Could you check a few things on this model? Use its own coordinates, in mm. A direction names the side the tool comes from. Round coordinates to 2 decimals unless told otherwise and drop trailing zeros. Loops run counter-clockwise (first coordinate to the right, second up) from the corner with the lowest first, then second, coordinate; pieces in that order, holes last. Notation, with made-up numbers: (15.25, -4) - (47.25, -4) arc R25 ccw to (47.25, 32) - close; hole circle Ø2 at (13, 89.5). An arc over 180 degrees is marked (long way). Use one line per item in the form item = value.
```python
from build123d import *

# Parameters (mm, degrees)
SKETCH1_W           = 5.6
SKETCH1_H           = 10
BOSS_EXTRUDE1_DEPTH = 4.5
CHAMFER1_SIZE       = 1
SKETCH2_R           = 1.5
BOSS_EXTRUDE2_DEPTH = 0.9
SKETCH3_W           = 3.6
SKETCH3_H           = 0.5
BOSS_EXTRUDE3_DEPTH = 2.4
CHAMFER2_SIZE       = 0.5


# Read off the part's stored shape, not the designer's step: Dome1, Dome2
with BuildPart() as part:
    # Sketch1 → Boss-Extrude1 (new body)
    with BuildSketch(Plane.XY):
        Rectangle(SKETCH1_W, SKETCH1_H)
    extrude(amount=BOSS_EXTRUDE1_DEPTH)

    # Chamfer1
    chamfer1_edges = [part.edges().sort_by_distance(p)[0] for p in [
        (-2.8, 0, 4.5),
        (0, -5, 4.5),
        (2.8, 0, 4.5),
        (0, 5, 4.5),
        (2.8, -5, 2.25),
        (-2.8, -5, 2.25),
    ]]
    chamfer(chamfer1_edges, length=CHAMFER1_SIZE)

    # Sketch2 → Boss-Extrude2 (add)
    with BuildSketch(Plane.XY.offset(4.5)):
        with Locations((0, 1.85)):
            Circle(SKETCH2_R)
        with Locations((0, -1.85)):
            Circle(SKETCH2_R)
    extrude(amount=BOSS_EXTRUDE2_DEPTH)

    # Dome1 outline → Dome1 (revolve)
    with BuildSketch(Plane.XZ.offset(-1.85)):
        with BuildLine():
            Line((0, 5.4), (1.5, 5.399999999))
            ThreePointArc((1.5, 5.399999999), (1.025914227, 6.395622385), (0, 6.8))
            Line((0, 6.8), (0, 5.4))
        make_face()
    revolve(axis=Axis((0, 1.85, 0), (0, 0, 1)))

    # Dome2 outline → Dome2 (revolve)
    with BuildSketch(Plane.XZ.offset(1.85)):
        with BuildLine():
            Line((0, 5.4), (1.5, 5.399999999))
            ThreePointArc((1.5, 5.399999999), (1.025914227, 6.395622385), (0, 6.8))
            Line((0, 6.8), (0, 5.4))
        make_face()
    revolve(axis=Axis((0, -1.85, 0), (0, 0, 1)))

    # Sketch3 → Boss-Extrude3 (add)
    with BuildSketch(Plane.XY.offset(4.5)):
        Rectangle(SKETCH3_W, SKETCH3_H)
    extrude(amount=BOSS_EXTRUDE3_DEPTH)

    # Chamfer2
    chamfer2_edges = [part.edges().sort_by_distance(p)[0] for p in [
        (1.8, 0, 6.9),
        (-1.8, 0, 6.9),
    ]]
    chamfer(chamfer2_edges, length=CHAMFER2_SIZE)


solid = part.part
```
1. If we section it at A-A, the plane z = 5: Write out the boundary of the cut face in (x, y), plus the area to 3 significant figures.
Solution:
outline = (-1.8, -0.25) - (1.8, -0.25) - (1.8, 0.25) - (-1.8, 0.25) - close; circle Ø3 at (0, -1.85); circle Ø3 at (0, 1.85)
area = 15.9 mm^2
2. We'd pull the mould along Y, two halves only. Please class faces 4 (the face through (0, -5, 2)), 5 (the face through (-1.5, 1.9, 4.9)), 6 (the face through (2.3, 0.4, 4)), 7 (the face through (-0.8, 3.4, 4.5)): +Y half, -Y half, draft (parallel to the pull), parting line (faces both ways), or undercut.
Solution:
face_4 = -Y half
face_5 = undercut
face_6 = draft
face_7 = undercut
3. If we section it at C-C, the plane y = -1.85: Write out the boundary of the cut face in (x, z).
Solution:
outline = (-2.8, 0) - (2.8, 0) - (2.8, 3.5) - (1.8, 4.5) - (1.5, 4.5) - (1.5, 5.4) arc R1.5 ccw to (-1.5, 5.4) - (-1.5, 4.5) - (-1.8, 4.5) - (-2.8, 3.5) - close
4. For P1, Ø2.5, axis at x = 0.5, z = 5.5, coming from the +Y side; P2, Ø3, axis at x = -0.5, y = 2, coming from the +Z side; P3, Ø2, axis at x = -1, z = 6, coming from the -Y side, each with a flat end and sliding along its axis, tell me the tip position at first contact or that it passes through.
Solution:
P1 = 4.25
P2 = 6.8
P3 = -3.34
5. On a 3-axis mill with a long thin cutter (end or side, diameter ignored), from which of +Z, -Z, +X, -X, +Y, -Y can I reach the whole of each face in a straight line? I mean faces 1 (the face through (-0.325, -3.314, 4.944)), 2 (the face through (-2.3, 0.4, 4)), 3 (the face through (0, -0.25, 6)). Say none if no direction works.
Solution:
face_1 = +Z
face_2 = +Z, -X, +Y, -Y
face_3 = +Z, +X, -X
6. If we section it at D-D, the plane z = 4: Write out the boundary of the cut face in (x, y), plus the area to 4 significant figures.
Solution:
outline = (-2.3, -4) - (-1.8, -4.5) - (1.8, -4.5) - (2.3, -4) - (2.3, 4.5) - (-2.3, 4.5) - close
area = 41.15 mm^2
7. Please list where these lines run through material, in increasing order: line 1 along Z through (x, y) = (2.3, 0); line 2 along Z through (x, y) = (-0.15, 3.75); line 3 along X through (y, z) = (-1.25, 5).
Solution:
line_1 = 0 to 4
line_2 = 0 to 4.5
line_3 = -1.37 to 1.37
